```python
from build123d import *

# Parameters (mm, degrees)
BOSS_EXTRUDE1_DEPTH      = 20.5
BOSS_EXTRUDE1_DEPTH_BACK = 20.5
SKETCH1_R                = 35
SKETCH1_R_2              = 32
SKETCH5_R                = 12.25
CUT_EXTRUDE2_DEPTH       = 54.574714185
SKETCH6_R                = 12.25
CUT_EXTRUDE3_DEPTH       = 54.574714354


with BuildPart() as part:
    # Sketch1 → Boss-Extrude1 (new, two sides: drawn at the far end of the back side and taken through both)
    with BuildSketch(Plane.XY.offset(-BOSS_EXTRUDE1_DEPTH_BACK)):
        Circle(SKETCH1_R)
        Circle(SKETCH1_R_2, mode=Mode.SUBTRACT)
    extrude(amount=BOSS_EXTRUDE1_DEPTH + BOSS_EXTRUDE1_DEPTH_BACK)

    # Sketch5 → Cut-Extrude2 (cut, through all)
    with BuildSketch(Plane(origin=(0, 0, 0), x_dir=(0, 0, -1), z_dir=(1, 0, 0))):
        Circle(SKETCH5_R)
    extrude(amount=-CUT_EXTRUDE2_DEPTH, mode=Mode.SUBTRACT)

    # Sketch6 → Cut-Extrude3 (cut, through all)
    with BuildSketch(Plane(origin=(0, 0, 0), x_dir=(1, 0, 0), z_dir=(0, 1, 0))):
        with Locations(Location((0, 0, 0), (0, 0, 270))):
            Circle(SKETCH6_R)
    extrude(amount=-CUT_EXTRUDE3_DEPTH, mode=Mode.SUBTRACT)


solid = part.part
```
Geometry check sheet. Reference: the model listing, model coordinates, mm. A direction names the side the tool comes from. Round coordinates to 2 decimals unless told otherwise and drop trailing zeros. Loops run counter-clockwise (first coordinate to the right, second up) from the corner with the lowest first, then second, coordinate; pieces in that order, holes last. Notation, with made-up numbers: (11, -30) - (54, -30) arc R21 cw to (54, -26) - close; hole circle Ø10 at (72.5, 30.5). An arc over 180 degrees is marked (long way). Use a Markdown table: item, result.
Q1. Access from +Z, -Z, +X, -X, +Y, -Y to the whole of each face (thin tool, end or side, straight path). Record for faces 4 (the cylindrical face through (30.522, 9.612, -0.287)), 5 (the cylindrical face through (-32.243, -11.959, 2.656)).
Solutions:
| item | result |
|---|---|
| face 4 | +Z, -Z |
| face 5 | -X |
Q2. Draft check along X on faces 1 (the flat face through (15.4, -28.4, -20.5)), 2 (the cylindrical face through (-11.959, -32.243, -2.656)), 3 (the cylindrical face through (33.384, 10.513, -0.287)). Enter one of: released by +X, released by -X, zero draft, split by the parting line, or undercut.
Solutions:
| item | result |
|---|---|
| face 1 | zero draft |
| face 2 | undercut |
| face 3 | split by the parting line |
Q3. Cross-section at D-D on y = -31. Record the cut outline in (x, z).
Solutions:
| item | result |
|---|---|
| outline | (-16.25, -20.5) - (-7.94, -20.5) - (-7.94, -9.33) arc R12.25 cw to (-7.94, 9.33) - (-7.94, 20.5) - (-16.25, 20.5) - close; (7.94, -20.5) - (16.25, -20.5) - (16.25, 20.5) - (7.94, 20.5) - (7.94, 9.33) arc R12.25 cw to (7.94, -9.33) - close |
Q4. Cross-section at C-C on z = 10. Record the cut outline in (x, y).
Solutions:
| item | result |
|---|---|
| outline | (-34.28, -7.08) arc R35 ccw to (-7.08, -34.28) - (-7.08, -31.21) arc R32 cw to (-31.21, -7.08) - close; (-34.28, 7.08) - (-31.21, 7.08) arc R32 cw (long way) to (7.08, -31.21) - (7.08, -34.28) arc R35 ccw (long way) to start |
Q5. Go/stop test with flat-tipped pins: P1, Ø12, axis at y = -27, z = 1, coming from the +X side; P2, Ø4, axis at y = -4, z = 6.5, coming from the -X side; P3, Ø1, axis at x = -19, z = -11, coming from the -Y side. Record where each tip stops, or that it passes through.
Solutions:
| item | result |
|---|---|
| P1 | stops at x = 28 |
| P2 | stops at x = 31.43 |
| P3 | stops at y = -29.71 |
Q6. Material ranges on line 1 (Z direction, x = 0, y = -33); line 2 (Y direction, x = -31.65, z = 0); line 3 (Y direction, x = -31, z = 2.5), recorded low to high.
Solutions:
| item | result |
|---|---|
| line 1 | z = -20.5 to -12.25, 12.25 to 20.5 |
| line 2 | y = -14.94 to -12.25, 12.25 to 14.94 |
| line 3 | y = -16.25 to -11.99, 11.99 to 16.25 |
Q7. Cross-section at A-A on x = 0. Record the cut outline in (y, z).
Solutions:
| item | result |
|---|---|
| outline | (-35, -20.5) - (-32, -20.5) - (-32, -12.25) - (-35, -12.25) - close; (-35, 12.25) - (-32, 12.25) - (-32, 20.5) - (-35, 20.5) - close; (32, -20.5) - (35, -20.5) - (35, 20.5) - (32, 20.5) - close |
